Input: part model. Units: mm. Frame: model coordinates. A direction names the side the tool comes from. Give positions to 0.01 mm unless a question says otherwise; leave off trailing zeros. Write each loop counter-clockwise with the first axis right and the second up, starting at its lowest first coordinate (ties: lowest second). Pieces come first, ordered by that corner, then holes. Notation, with made-up numbers: (34, 7.5) - (61, 7.5) arc R11 ccw to (61, 27.5) - close; hole circle Ø9 at (77.5, 64.25). An arc over 180 degrees is marked (long way). Answer as CSV lines item,"result".
```python
from build123d import *

# Parameters (mm, degrees)
BOSS_EXTRUDE1_DEPTH   = 63
BOSS_EXTRUDE1_2_DEPTH = 63
BOSS_EXTRUDE2_START   = -12
BOSS_EXTRUDE2_DEPTH   = 51
BOSS_EXTRUDE3_START   = -19
BOSS_EXTRUDE3_DEPTH   = 25
BOSS_EXTRUDE4_START   = -41
BOSS_EXTRUDE4_DEPTH   = 22
BOSS_EXTRUDE5_DEPTH   = 22


with BuildPart() as part:
    # Sketch1 → Boss-Extrude1 (new body)
    with BuildSketch(Plane.XY):
        Polygon((-75, 0), (-50, 0), (-50, 24.666666667), (-63, 18.08), (-75, 12), align=None)
    extrude(amount=-BOSS_EXTRUDE1_DEPTH)



with BuildPart() as body_2:
    # Sketch1 → Boss-Extrude1 2 (new body)
    with BuildSketch(Plane.XY):
        Polygon((-25, 0), (0, 0), (0, 38), (-23.684210526, 38), (-25, 37.333333333), align=None)
    extrude(amount=-BOSS_EXTRUDE1_2_DEPTH)


with BuildPart() as part_1:
    add(part.part)

    add(body_2.part)  # Boss-Extrude2 merges body 2
    # Sketch1_3 → Boss-Extrude2 (add)
    with BuildSketch(Plane.XY.offset(BOSS_EXTRUDE2_START)):
        Polygon((-50, 0), (-25, 0), (-25, 37.333333333), (-31.421052632, 34.08), (-50, 24.666666667), align=None)
    extrude(amount=-BOSS_EXTRUDE2_DEPTH)

    # Sketch1_4 → Boss-Extrude3 (add)
    with BuildSketch(Plane.XY.offset(BOSS_EXTRUDE3_START)):
        Polygon((-63, 18.08), (-50, 24.666666667), (-31.421052632, 34.08), (-63, 34.08), align=None)
    extrude(amount=-BOSS_EXTRUDE3_DEPTH)

    # Sketch1_5 → Boss-Extrude4 (add)
    with BuildSketch(Plane.XY.offset(BOSS_EXTRUDE4_START)):
        Polygon((-23.684210526, 38), (0, 38), (0, 50), align=None)
    extrude(amount=-BOSS_EXTRUDE4_DEPTH)

    # Sketch1_6 → Boss-Extrude5 (add)
    with BuildSketch(Plane.XY):
        Polygon((-23.684210526, 38), (0, 38), (0, 50), align=None)
    extrude(amount=-BOSS_EXTRUDE5_DEPTH)


solid = part_1.part
```
Item 1: Cut plane C-C on z = -38. Return the cut outline in (x, y).
The answers:
outline,"(-75, 0) - (0, 0) - (0, 38) - (-23.68, 38) - (-31.42, 34.08) - (-63, 34.08) - (-63, 18.08) - (-75, 12) - close"
Item 2: Cut plane D-D on x = -36. Return the cut outline in (y, z).
The answers:
outline,"(0, -63) - (31.76, -63) - (31.76, -44) - (34.08, -44) - (34.08, -19) - (31.76, -19) - (31.76, -12) - (0, -12) - close"
Item 3: Contact query for flat-ended pins moving along their axis: pin 1 (8 mm diameter, centred on x = -32, z = -16.5, fed in from +Y); pin 2 (3.5 mm diameter, centred on y = 19, z = -7, fed in from -X); pin 3 (5 mm diameter, centred on y = 27.5, z = -26, fed in from -X); pin 4 (6 mm diameter, centred on x = -57.5, y = 37.5, fed in from -Z). Output: stop coordinate, or through.
The answers:
pin 1,"y = 35.81"
pin 2,"x = -64.64"
pin 3,"x = -63"
pin 4,"through"
Item 4: Reachability of faces 5 (the face through (-25, 19, -6)), 6 (the face through (-7, 41, -41)), 7 (the face through (-51, 28, -44)), 8 (the face through (-63, 26, -31)), 9 (the face through (-51, 28, -19)) from +Z, -Z, +X, -X, +Y, -Y: full face, straight path, thin tool, end or side. Return the list, or none.
The answers:
face 5,"+Z, +Y, -Y"
face 6,"+X, -X, +Y"
face 7,"-Z, -X, +Y"
face 8,"+Z, -Z, -X, +Y"
face 9,"+Z, -X, +Y"
Item 5: Cut plane A-A on z = -5. Return the cut outline in (x, y), plus the area to 3 significant figures.
The answers:
outline,"(-75, 0) - (-50, 0) - (-50, 24.67) - (-75, 12) - close; (-25, 0) - (0, 0) - (0, 50) - (-25, 37.33) - close"
area,"1,550 mm²"
Item 6: Cut plane B-B on y = 44.5. Return the cut outline in (x, z), plus the area to 3 significant figures.
The answers:
outline,"(-10.86, -63) - (0, -63) - (0, -41) - (-10.86, -41) - close; (-10.86, -22) - (0, -22) - (0, 0) - (-10.86, 0) - close"
area,"478 mm²"
Item 7: Mould query, pull axis Z, two halves, no side actions, for faces 1 (the face through (-12, 38, -31)), 2 (the face through (-47, 34.08, -31)), 3 (the face through (-7, 41, -22)), 4 (the face through (-63, 10, 0)). Classes: +Z half, -Z half, draft (parallel to the pull), parting line (faces both ways), or undercut.
The answers:
face 1,"undercut"
face 2,"draft"
face 3,"undercut"
face 4,"+Z half"
Item 8: Ray query, line 1 (X direction, y = 31.5, z = -37); line 2 (Y direction, x = -10, z = -37.5); line 3 (Z direction, x = -38.5, y = 23.5). Return the intervals inside material, ascending. Write a range as from..to.
The answers:
line 1,"-63..0"
line 2,"0..38"
line 3,"-63..-12"
